```python
from build123d import *

# Parameters (mm, degrees)
SKETCH_2_W             = 160
SKETCH_2_H             = 250
EXTRUDE_295_DEPTH      = 5
SKETCH_6_R             = 1.6
CUT_EXTRUDE_1846_DEPTH = 297.858552176
SKETCH_7_R             = 1.6
L298N_DEPTH            = 297.858552176
SKETCH_9_R             = 1.6
CUT_EXTRUDE_3042_DEPTH = 10
SKETCH_10_R            = 1.6
CUT_EXTRUDE_3635_DEPTH = 297.858552176
SKETCH_11_W            = 45
SKETCH_11_H            = 60
CUT_EXTRUDE_2560_DEPTH = 297.858552176
SKETCH_12_R            = 1.6
CUT_EXTRUDE_2_DEPTH    = 297.858552176
EXTRUDE_1_DEPTH        = 5
SKETCH_14_W            = 42
SKETCH_14_H            = 120
EXTRUDE_2_DEPTH        = 5
SKETCH_15_W            = 7
SKETCH_15_H            = 90
EXTRUDE_3_DEPTH        = 5


with BuildPart() as part:
    # 草图2 → Extrude 295 (new body)
    with BuildSketch(Plane(origin=(0, 0, 0), x_dir=(1, 0, 0), z_dir=(0, 1, 0))):
        with Locations((80, 125)):
            Rectangle(SKETCH_2_W, SKETCH_2_H)
    extrude(amount=EXTRUDE_295_DEPTH)

    # 草图6 → Cut-Extrude 1846 (cut, through all)
    with BuildSketch(Plane(origin=(0, 5, 0), x_dir=(1, 0, 0), z_dir=(0, 1, 0))):
        with Locations(Location((8, 245, 0), (0, 0, 270))):
            Circle(SKETCH_6_R)
        with Locations(Location((32, 245, 0), (0, 0, 270))):
            Circle(SKETCH_6_R)
        with Locations(Location((8, 215, 0), (0, 0, 270))):
            Circle(SKETCH_6_R)
        with Locations(Location((32, 215, 0), (0, 0, 270))):
            Circle(SKETCH_6_R)
        with Locations(Location((128, 245, 0), (0, 0, 270))):
            Circle(SKETCH_6_R)
        with Locations(Location((152, 245, 0), (0, 0, 270))):
            Circle(SKETCH_6_R)
        with Locations(Location((128, 215, 0), (0, 0, 270))):
            Circle(SKETCH_6_R)
        with Locations(Location((152, 215, 0), (0, 0, 270))):
            Circle(SKETCH_6_R)
        with Locations(Location((32, 35, 0), (0, 0, 270))):
            Circle(SKETCH_6_R)
        with Locations(Location((8, 35, 0), (0, 0, 270))):
            Circle(SKETCH_6_R)
        with Locations(Location((8, 5, 0), (0, 0, 270))):
            Circle(SKETCH_6_R)
        with Locations(Location((32, 5, 0), (0, 0, 270))):
            Circle(SKETCH_6_R)
        with Locations(Location((128, 35, 0), (0, 0, 270))):
            Circle(SKETCH_6_R)
        with Locations(Location((152, 35, 0), (0, 0, 270))):
            Circle(SKETCH_6_R)
        with Locations(Location((128, 5, 0), (0, 0, 270))):
            Circle(SKETCH_6_R)
        with Locations(Location((152, 5, 0), (0, 0, 270))):
            Circle(SKETCH_6_R)
    extrude(amount=-CUT_EXTRUDE_1846_DEPTH, mode=Mode.SUBTRACT)

    # 草图7 → L298N固定 (cut, through all)
    with BuildSketch(Plane(origin=(0, 5, 0), x_dir=(1, 0, 0), z_dir=(0, 1, 0))):
        with Locations(Location((3, 110, 0), (0, 0, 270))):
            Circle(SKETCH_7_R)
        with Locations(Location((40, 73, 0), (0, 0, 270))):
            Circle(SKETCH_7_R)
        with Locations(Location((3, 73, 0), (0, 0, 270))):
            Circle(SKETCH_7_R)
        with Locations(Location((40, 110, 0), (0, 0, 270))):
            Circle(SKETCH_7_R)
        with Locations(Location((120, 110, 0), (0, 0, 270))):
            Circle(SKETCH_7_R)
        with Locations(Location((157, 73, 0), (0, 0, 270))):
            Circle(SKETCH_7_R)
        with Locations(Location((120, 73, 0), (0, 0, 270))):
            Circle(SKETCH_7_R)
        with Locations(Location((157, 110, 0), (0, 0, 270))):
            Circle(SKETCH_7_R)
    extrude(amount=-L298N_DEPTH, mode=Mode.SUBTRACT)

    # 草图9 → Cut-Extrude 3042 (cut)
    with BuildSketch(Plane.XZ):
        with Locations(Location((36.5, -195, 0), (0, 0, 270))):
            Circle(SKETCH_9_R)
        with Locations(Location((10, -136, 0), (0, 0, 270))):
            Circle(SKETCH_9_R)
        with Locations(Location((10, -195, 0), (0, 0, 270))):
            Circle(SKETCH_9_R)
        with Locations(Location((36.5, -136, 0), (0, 0, 270))):
            Circle(SKETCH_9_R)
    extrude(amount=-CUT_EXTRUDE_3042_DEPTH, mode=Mode.SUBTRACT)

    # 草图10 → Cut-Extrude 3635 (cut, through all)
    with BuildSketch(Plane.XZ):
        with Locations(Location((40, -123, 0), (0, 0, 270))):
            Circle(SKETCH_10_R)
        with Locations(Location((120, -123, 0), (0, 0, 270))):
            Circle(SKETCH_10_R)
        with Locations(Location((40, -58, 0), (0, 0, 270))):
            Circle(SKETCH_10_R)
        with Locations(Location((120, -58, 0), (0, 0, 270))):
            Circle(SKETCH_10_R)
    extrude(amount=-CUT_EXTRUDE_3635_DEPTH, mode=Mode.SUBTRACT)

    # 草图11 → Cut-Extrude 2560 (cut, through all)
    with BuildSketch(Plane(origin=(0, 5, 0), x_dir=(1, 0, 0), z_dir=(0, 1, 0))):
        with Locations((80, 40)):
            Rectangle(SKETCH_11_W, SKETCH_11_H)
    extrude(amount=-CUT_EXTRUDE_2560_DEPTH, mode=Mode.SUBTRACT)

    # 草图12 → 切除-拉伸2 (cut, through all)
    with BuildSketch(Plane(origin=(0, 5, 0), x_dir=(1, 0, 0), z_dir=(0, 1, 0))):
        with Locations(Location((106.5, 13, 0), (0, 0, 270))):
            Circle(SKETCH_12_R)
        with Locations(Location((53.5, 67, 0), (0, 0, 270))):
            Circle(SKETCH_12_R)
        with Locations(Location((106.5, 67, 0), (0, 0, 270))):
            Circle(SKETCH_12_R)
        with Locations(Location((53.5, 13, 0), (0, 0, 270))):
            Circle(SKETCH_12_R)
    extrude(amount=-CUT_EXTRUDE_2_DEPTH, mode=Mode.SUBTRACT)

    # 草图13 → 凸台-拉伸1 (add)
    with BuildSketch(Plane(origin=(0, 5, 0), x_dir=(1, 0, 0), z_dir=(0, 1, 0))):
        Polygon((202, -60), (-42, -60), (-42, -25), (0, -25), (0, 0), (160, 0), (160, -25), (202, -25), align=None)
        Polygon((202, 275), (160, 275), (160, 250), (0, 250), (0, 275), (-42, 275), (-42, 310), (202, 310), align=None)
    extrude(amount=-EXTRUDE_1_DEPTH)

    # 草图14 → 凸台-拉伸2 (add)
    with BuildSketch(Plane(origin=(0, 5, 0), x_dir=(1, 0, 0), z_dir=(0, 1, 0))):
        with Locations((181, 125)):
            Rectangle(SKETCH_14_W, SKETCH_14_H)
        with Locations((-21, 125)):
            Rectangle(SKETCH_14_W, SKETCH_14_H)
    extrude(amount=-EXTRUDE_2_DEPTH)

    # 草图15 → 凸台-拉伸3 (add)
    with BuildSketch(Plane(origin=(0, 5, 0), x_dir=(1, 0, 0), z_dir=(0, 1, 0))):
        with Locations((163.5, 20)):
            Rectangle(SKETCH_15_W, SKETCH_15_H)
        with Locations((163.5, 230)):
            Rectangle(SKETCH_15_W, SKETCH_15_H)
        with Locations((-3.5, 20)):
            Rectangle(SKETCH_15_W, SKETCH_15_H)
        with Locations((-3.5, 230)):
            Rectangle(SKETCH_15_W, SKETCH_15_H)
    extrude(amount=-EXTRUDE_3_DEPTH)


solid = part.part
```
Geometry check sheet. Reference: the model listing, model coordinates, mm. Round coordinates to 2 decimals unless told otherwise and drop trailing zeros. Loops run counter-clockwise (first coordinate to the right, second up) from the corner with the lowest first, then second, coordinate; pieces in that order, holes last. Notation, with made-up numbers: (52, 73.25) -> (87, 73.25) arc R22 cw to (87, 102.25) -> close; hole circle Ø5 at (86.5, 23.25). An arc over 180 degrees is marked (long way). Use a Markdown table: item, result.
(1) Sectioned sample at A-A (x = 72). Enter the section's corners in (y, z), then the cut area to 3 significant figures.
Calculated:
| item | result |
|---|---|
| outline | (0, -310) -> (5, -310) -> (5, -70) -> (0, -70) -> close; (0, -10) -> (5, -10) -> (5, 60) -> (0, 60) -> close |
| area | 1,550 mm² |
(2) Sectioned sample at B-B (z = 15.5). Enter the section's corners in (x, y).
Calculated:
| item | result |
|---|---|
| outline | (-7, 0) -> (167, 0) -> (167, 5) -> (-7, 5) -> close |
(3) Go/stop test with flat-tipped pins: P1, Ø1.5, axis at y = 2, z = -42, coming from the -X side; P2, Ø2.5, axis at y = 3, z = -227.5, coming from the +X side. Record where each tip stops, or that it passes through.
Calculated:
| item | result |
|---|---|
| P1 | x = -7 |
| P2 | x = 167 |
(4) Sectioned sample at C-C (y = 3.6). Give the number of separate pieces and of enclosed holes in the cut face, then the cut area to 3 significant figures.
Calculated:
| item | result |
|---|---|
| separate pieces | 1 |
| enclosed holes | 37 |
| area | 74,700 mm² |
(5) Scan lines: probe 1 along Z at (x, y) = (-26, 2.45); probe 2 along X at (y, z) = (2.1, -67); probe 3 along X at (y, z) = (1.45, -245). Record each from-to range of solid material in increasing order.
Calculated:
| item | result |
|---|---|
| probe 1 | -310 to -275, -185 to -65, 25 to 60 |
| probe 2 | -42 to 51.9, 55.1 to 57.5, 102.5 to 104.9, 108.1 to 202 |
| probe 3 | -7 to 6.4, 9.6 to 30.4, 33.6 to 126.4, 129.6 to 150.4, 153.6 to 167 |
